Input: part model. Units: mm. Frame: model coordinates. Face numbers are marked on the shaded views. A direction names the side the tool comes from. Coordinates: 2 decimals unless noted, no trailing zeros. Write each loop counter-clockwise with the first axis right and the second up, starting at its lowest first coordinate (ties: lowest second). Pieces come first, ordered by that corner, then holes. Notation, with made-up numbers: M -15.75,-29.5 L 25.25,-29.5 A24 ccw 25.25,-15.5 Z; hole C 70.25,-19.75 d2. An arc over 180 degrees is marked long. Answer as a JSON object with one key per item and string values. Group by question number.
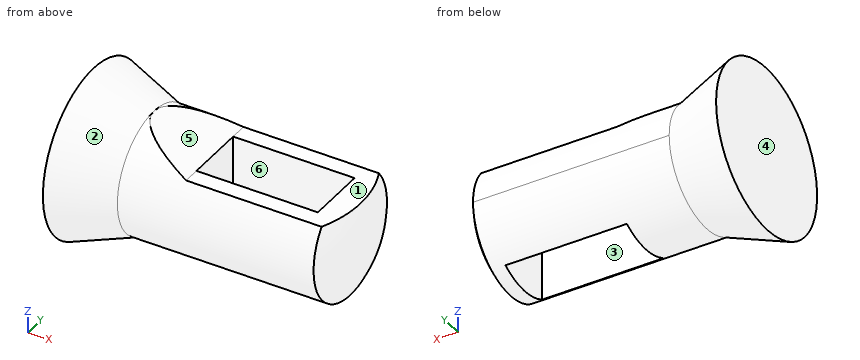
from build123d import *

# Parameters (mm, degrees)
CUT_EXTRUDE2_DEPTH      = 35.925
CUT_EXTRUDE2_DEPTH_BACK = 35.925
SKETCH4_W               = 50.8
SKETCH4_H               = 25.4
CUT_EXTRUDE3_DEPTH      = 51.8


with BuildPart() as part:
    # Sketch1 → Revolve1 (revolve)
    with BuildSketch(Plane.XY):
        with BuildLine():
            Line((0, 0), (0, 34.925))
            Line((0, 34.925), (25.4, 25.4))
            Line((25.4, 25.4), (107.494090512, 25.4))
            ThreePointArc((107.494090512, 25.4), (112.569031975, 13.148007491), (114.3, 0))
            Line((114.3, 0), (0, 0))
        make_face()
    revolve(axis=Axis((0, 0, 0), (1, 0, 0)))

    # Sketch3 → Cut-Extrude2 (cut, two sides)
    with BuildSketch(Plane(origin=(0, 0, 0), x_dir=(1, 0, 0), z_dir=(0, 1, 0))) as cut_extrude2_sk:
        Polygon((25.4, -25.4), (50.8, -15.875), (114.3, -15.875), (114.3, -25.4), align=None)
    extrude(amount=CUT_EXTRUDE2_DEPTH, mode=Mode.SUBTRACT)
    extrude(cut_extrude2_sk.sketch, amount=-CUT_EXTRUDE2_DEPTH_BACK, mode=Mode.SUBTRACT)

    # Sketch4 → Cut-Extrude3 (cut, through all)
    with BuildSketch(Plane.XY.offset(15.875)):
        with Locations((76.2, 0)):
            Rectangle(SKETCH4_W, SKETCH4_H)
    extrude(amount=-CUT_EXTRUDE3_DEPTH, mode=Mode.SUBTRACT)


solid = part.part
Q1. Line query: line 1 (Y direction, x = 104, z = 1); line 2 (X direction, y = 10, z = -12); line 3 (Z direction, x = 82.5, y = 22). Output: solid intervals per line, ascending. Write a range as from..to.
Q2. Section A-A, the plane x = 81. Return the cut outline in (y, z) (3 decimals).
Q3. Draft query along X for the marked faces 1, 2, 3 and 4. Return one class per face: released by +X, released by -X, zero draft, split by the parting line, or undercut.
Q4. Access query for the marked faces 5 and 6. Directions: +Z, -Z, +X, -X, +Y, -Y. A direction counts if a zero-diameter tool reaches every point of the face in a straight line with its end or side. Return the directions, or none.
Q5. Section B-B, the plane x = 30. Return the cut outline in (y, z) (3 decimals), and give its area (3 significant figures).
Q6. Pin query (flat end, axial travel): pin 1 Ø10 at (x, z) = (76.5, -10.5) entering from +Y; pin 2 Ø5 at (x, y) = (49, -14) entering from +Z; pin 3 Ø8 at (x, z) = (97.5, -13.5) entering from -Y. Return the tip coordinate at first contact, or that it passes through.
Filled in:
{
 "1": {"line 1": "-25.38..25.38", "line 2": "0..50.8, 101.6..111.84", "line 3": "-12.69..12.69"},
 "2": {"outline": "M -19.828,15.875 A25.4 ccw -12.7,-21.997 L -12.7,15.875 Z; M 12.7,-21.997 A25.4 ccw 19.828,15.875 L 12.7,15.875 Z"},
 "3": {"face 1": "zero draft", "face 2": "released by +X", "face 3": "undercut", "face 4": "released by -X"},
 "4": {"face 5": "+Z, +X, +Y, -Y", "face 6": "+Z, -Z"},
 "5": {"outline": "M -9.201,23.675 A25.4 ccw long 9.201,23.675 Z", "area": "2,010 mm^2"},
 "6": {"pin 1": "y = 24.8", "pin 2": "z = 17.49", "pin 3": "y = -23.56"}
}
